Could you check a few things on this model? Use its own coordinates, in mm. Face numbers are marked on the shaded views. A direction names the side the tool comes from. Round coordinates to 2 decimals unless told otherwise and drop trailing zeros. Loops run counter-clockwise (first coordinate to the right, second up) from the corner with the lowest first, then second, coordinate; pieces in that order, holes last. Notation, with made-up numbers: (83.5, 87) -> (129.5, 87) arc R22 cw to (129.5, 98) -> close; hole circle Ø3 at (-26.5, 31.5). An arc over 180 degrees is marked (long way). One line per item, written item: value.
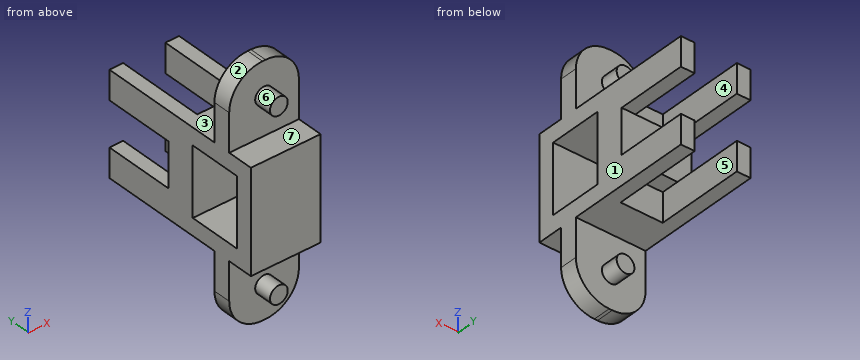
```python
from build123d import *

# Parameters (mm, degrees)
SKETCH4_W               = 31.4
SKETCH4_H               = 31.4
SKETCH4_W_2             = 25.4
SKETCH4_H_2             = 25.4
BOSS_EXTRUDE3_DEPTH     = 30
SKETCH5_W               = 31.4
SKETCH5_H               = 31.4
BOSS_EXTRUDE4_DEPTH     = 5
SKETCH6_W               = 31.4
SKETCH6_H               = 8
BOSS_EXTRUDE5_DEPTH     = 5
BOSS_EXTRUDE6_DEPTH     = 8
SKETCH8_R               = 4
BOSS_EXTRUDE7_DEPTH     = 8
SKETCH9_W               = 31.4
SKETCH9_H               = 10
BOSS_EXTRUDE8_DEPTH     = 5
SKETCH10_W              = 31.4
SKETCH10_H              = 10
BOSS_EXTRUDE9_DEPTH     = 13
SKETCH11_W              = 6.2
SKETCH11_H              = 10
BOSS_EXTRUDE10_DEPTH    = 40
BOSS_EXTRUDE11_DEPTH    = 3
SKETCH13_W              = 31.4
SKETCH13_H              = 31.4
CUT_EXTRUDE1_DEPTH      = 31.4
SKETCH14_W              = 31.4
SKETCH14_H              = 31.4
BOSS_EXTRUDE12_DEPTH    = 4
SKETCH16_W              = 31.4
SKETCH16_H              = 8
BOSS_EXTRUDE13_DEPTH    = 15.4
MIRROR2_COPY_1_SKETCH_R = 4
MIRROR2_COPY_1_DEPTH    = 8
SKETCH17_W              = 30.8
SKETCH17_H              = 24
CUT_EXTRUDE2_DEPTH      = 31.4


with BuildPart() as part:
    # Sketch4 → Boss-Extrude3 (new body)
    with BuildSketch(Plane.XY):
        Rectangle(SKETCH4_W, SKETCH4_H)
        Rectangle(SKETCH4_W_2, SKETCH4_H_2, mode=Mode.SUBTRACT)
    boss_extrude3 = extrude(amount=BOSS_EXTRUDE3_DEPTH)

    # Sketch5 → Boss-Extrude4 (add)
    with BuildSketch(Plane.XY.offset(30)):
        Rectangle(SKETCH5_W, SKETCH5_H)
    boss_extrude4 = extrude(amount=BOSS_EXTRUDE4_DEPTH)

    # Sketch6 → Boss-Extrude5 (add)
    with BuildSketch(Plane.XY.offset(35)):
        Rectangle(SKETCH6_W, SKETCH6_H)
    boss_extrude5 = extrude(amount=BOSS_EXTRUDE5_DEPTH)

    # Sketch7 → Boss-Extrude6 (add)
    with BuildSketch(Plane.XZ.offset(4)):
        with BuildLine():
            Line((-15.7, 40), (-15.7, 52))
            ThreePointArc((-15.7, 52), (-11.306601718, 62.606601718), (-0.7, 67))
            Line((-0.7, 67), (0.7, 67))
            ThreePointArc((0.7, 67), (11.306601718, 62.606601718), (15.7, 52))
            Line((15.7, 52), (15.7, 40))
            Line((15.7, 40), (-15.7, 40))
        make_face()
    boss_extrude6 = extrude(amount=-BOSS_EXTRUDE6_DEPTH)

    # Sketch8 → Boss-Extrude7 (add)
    with BuildSketch(Plane.XZ.offset(4)):
        with Locations(Location((0, 52, 0), (0, 0, 180))):
            Circle(SKETCH8_R)
    boss_extrude7 = extrude(amount=BOSS_EXTRUDE7_DEPTH)

    # Mirror1: Boss-Extrude7 across plane
    add(boss_extrude7.mirror(Plane.ZX))

    # Sketch9 → Boss-Extrude8 (add)
    with BuildSketch(Plane(origin=(0, 15.7, 0), x_dir=(1, 0, 0), z_dir=(0, 1, 0))):
        with Locations((0, -27)):
            Rectangle(SKETCH9_W, SKETCH9_H)
    boss_extrude8 = extrude(amount=BOSS_EXTRUDE8_DEPTH)

    # Sketch10 → Boss-Extrude9 (add)
    with BuildSketch(Plane(origin=(0, 15.7, 0), x_dir=(1, 0, 0), z_dir=(0, 1, 0))):
        with Locations((0, -17)):
            Rectangle(SKETCH10_W, SKETCH10_H)
    boss_extrude9 = extrude(amount=BOSS_EXTRUDE9_DEPTH)

    # Sketch11 → Boss-Extrude10 (add)
    with BuildSketch(Plane(origin=(0, 20.7, 0), x_dir=(1, 0, 0), z_dir=(0, 1, 0))):
        with Locations((-12.6, -27)):
            Rectangle(SKETCH11_W, SKETCH11_H)
        with Locations((12.6, -27)):
            Rectangle(SKETCH11_W, SKETCH11_H)
    boss_extrude10 = extrude(amount=BOSS_EXTRUDE10_DEPTH)

    # Sketch12 → Boss-Extrude11 (add)
    with BuildSketch(Plane.XY.offset(32)):
        Polygon((-15.7, 60.7), (-9.5, 60.7), (-9.5, 20.7), (9.5, 20.7), (9.5, 60.7), (15.7, 60.7), (15.7, 15.7), (-15.7, 15.7), align=None)
    boss_extrude11 = extrude(amount=BOSS_EXTRUDE11_DEPTH)

    # Sketch13 → Cut-Extrude1 (cut)
    with BuildSketch(Plane.ZY.offset(15.7)):
        with Locations((15.7, 0)):
            Rectangle(SKETCH13_W, SKETCH13_H)
    extrude(amount=-CUT_EXTRUDE1_DEPTH, mode=Mode.SUBTRACT)

    # Sketch14 → Boss-Extrude12 (add)
    with BuildSketch(Plane(origin=(0, 0, 31.4), x_dir=(-1, 0, 0), z_dir=(0, 0, -1))):
        Rectangle(SKETCH14_W, SKETCH14_H)
    boss_extrude12 = extrude(amount=BOSS_EXTRUDE12_DEPTH)

    # Sketch16 → Boss-Extrude13 (add)
    with BuildSketch(Plane(origin=(0, 0, 27.4), x_dir=(-1, 0, 0), z_dir=(0, 0, -1))):
        with Locations((0, -11.7)):
            Rectangle(SKETCH16_W, SKETCH16_H)
    boss_extrude13 = extrude(amount=BOSS_EXTRUDE13_DEPTH)

    # Mirror2: Boss-Extrude3, Boss-Extrude4, Boss-Extrude5, Boss-Extrude6, Boss-Extrude7, Boss-Extrude8, Boss-Extrude9, Boss-Extrude10, Boss-Extrude11, Boss-Extrude12, Boss-Extrude13 across plane
    add(boss_extrude3.mirror(Plane(origin=(-15.7, 28.7, 12), x_dir=(1, 0, 0), z_dir=(0, 0, 1))))
    add(boss_extrude4.mirror(Plane(origin=(-15.7, 28.7, 12), x_dir=(1, 0, 0), z_dir=(0, 0, 1))))
    add(boss_extrude5.mirror(Plane(origin=(-15.7, 28.7, 12), x_dir=(1, 0, 0), z_dir=(0, 0, 1))))
    add(boss_extrude6.mirror(Plane(origin=(-15.7, 28.7, 12), x_dir=(1, 0, 0), z_dir=(0, 0, 1))))
    add(boss_extrude7.mirror(Plane(origin=(-15.7, 28.7, 12), x_dir=(1, 0, 0), z_dir=(0, 0, 1))))
    add(boss_extrude8.mirror(Plane(origin=(-15.7, 28.7, 12), x_dir=(1, 0, 0), z_dir=(0, 0, 1))))
    add(boss_extrude9.mirror(Plane(origin=(-15.7, 28.7, 12), x_dir=(1, 0, 0), z_dir=(0, 0, 1))))
    add(boss_extrude10.mirror(Plane(origin=(-15.7, 28.7, 12), x_dir=(1, 0, 0), z_dir=(0, 0, 1))))
    add(boss_extrude11.mirror(Plane(origin=(-15.7, 28.7, 12), x_dir=(1, 0, 0), z_dir=(0, 0, 1))))
    add(boss_extrude12.mirror(Plane(origin=(-15.7, 28.7, 12), x_dir=(1, 0, 0), z_dir=(0, 0, 1))))
    add(boss_extrude13.mirror(Plane(origin=(-15.7, 28.7, 12), x_dir=(1, 0, 0), z_dir=(0, 0, 1))))

    # Mirror2 copy 1 sketch → Mirror2 copy 1 (add)
    with BuildSketch(Plane(origin=(0, 4, 24), x_dir=(1, 0, 0), z_dir=(0, 1, 0))):
        with Locations(Location((0, 52, 0), (0, 0, 180))):
            Circle(MIRROR2_COPY_1_SKETCH_R)
    extrude(amount=MIRROR2_COPY_1_DEPTH)

    # Sketch17 → Cut-Extrude2 (cut)
    with BuildSketch(Plane.ZY.offset(15.7)):
        with Locations((12, 3.7)):
            Rectangle(SKETCH17_W, SKETCH17_H)
    extrude(amount=-CUT_EXTRUDE2_DEPTH, mode=Mode.SUBTRACT)


solid = part.part
```
(1) Imagine slicing it at B-B on y = 53. Write out the boundary of the cut face in (x, z), then the cut area to 3 significant figures.
Results below:
outline: (-15.7, -11) -> (-9.5, -11) -> (-9.5, 2) -> (-15.7, 2) -> close; (-15.7, 22) -> (-9.5, 22) -> (-9.5, 35) -> (-15.7, 35) -> close; (9.5, -11) -> (15.7, -11) -> (15.7, 2) -> (9.5, 2) -> close; (9.5, 22) -> (15.7, 22) -> (15.7, 35) -> (9.5, 35) -> close
area: 322 mm²
(2) Imagine slicing it at A-A on z = 18. Write out the boundary of the cut face in (x, y).
Results below:
outline: (-15.7, -15.7) -> (15.7, -15.7) -> (15.7, -8.3) -> (-15.7, -8.3) -> close; (-15.7, 15.7) -> (15.7, 15.7) -> (15.7, 28.7) -> (-15.7, 28.7) -> close
(3) Please list where these lines run through material, in increasing order: L1, parallel to Z at x = 13, y = 9; L2, parallel to X at y = 51, z = -4; L3, parallel to Y at x = -5.5, z = 1.5.
Results below:
L1: z = -11 to -3.4, 27.4 to 35
L2: x = -15.7 to -9.5, 9.5 to 15.7
L3: y = -15.7 to -8.3, 15.7 to 20.7
(4) We'd pull the mould along X, two halves only. Please class the marked faces 1, 2, 3 and 4: +X half, -X half, draft (parallel to the pull), parting line (faces both ways), or undercut.
Results below:
face 1: +X half
face 2: -X half
face 3: draft
face 4: undercut
(5) For pin 1 Ø15.5 at (x, y) = (6, 37.5) entering from +Z; pin 2 Ø4 at (x, y) = (0.5, 25.5) entering from -Z; pin 3 Ø9 at (x, z) = (2, 13.5) entering from +Y; pin 4 Ø12 at (x, y) = (-2.5, 40) entering from +Z, each with a flat end and sliding along its axis, tell me the tip position at first contact or that it passes through.
Results below:
pin 1: stops at z = 35
pin 2: stops at z = 2
pin 3: stops at y = 28.7
pin 4: passes through
(6) On a 3-axis mill with a long thin cutter (end or side, diameter ignored), from which of +Z, -Z, +X, -X, +Y, -Y can I reach the whole of each face in a straight line? I mean the marked faces 5, 6 and 7. Say none if no direction works.
Results below:
face 5: -Z, +Y
face 6: -Y
face 7: +X, -X, -Y
(7) Imagine slicing it at C-C on z = -9.5. Write out the boundary of the cut face in (x, y).
Results below:
outline: (-15.7, -15.7) -> (15.7, -15.7) -> (15.7, 60.7) -> (9.5, 60.7) -> (9.5, 20.7) -> (-9.5, 20.7) -> (-9.5, 60.7) -> (-15.7, 60.7) -> close
